```python
from build123d import *

# Parameters (mm, degrees)
BOSS_EXTRUDE1_DEPTH          = 4
BOSS_EXTRUDE1_DEPTH_BACK     = 1
SKETCH1_W                    = 120
SKETCH1_H                    = 120
FILLET1_R                    = 2.5
SKETCH34_W                   = 110
SKETCH34_H                   = 110
BOSS_EXTRUDE4_DEPTH          = 5
SKETCH35_W                   = 5
SKETCH35_H                   = 110
BOSS_EXTRUDE5_DEPTH          = 105
SKETCH36_W                   = 90
SKETCH36_H                   = 9.090388829
CUT_EXTRUDE17_DEPTH          = 5
F_97_0_0059_DIAMETER_HOLE2_D = 0.14986
F_1_0MM_DOWEL_HOLE1_D        = 1
SKETCH46_W                   = 17
SKETCH46_H                   = 15
CUT_EXTRUDE23_DEPTH          = 10
SKETCH50_W                   = 17
SKETCH50_H                   = 15
CUT_EXTRUDE24_DEPTH          = 10
SKETCH51_W                   = 17
SKETCH51_H                   = 15
CUT_EXTRUDE25_DEPTH          = 10
SKETCH52_W                   = 17
SKETCH52_H                   = 15
CUT_EXTRUDE26_DEPTH          = 10
SKETCH53_W                   = 0.977162156
SKETCH53_H                   = 13.998719243
BOSS_EXTRUDE6_DEPTH          = 5
SKETCH55_W                   = 2.272024092
SKETCH55_H                   = 13.774773728
CUT_EXTRUDE27_DEPTH          = 5
SKETCH56_W                   = 0.906735868
SKETCH56_H                   = 14
BOSS_EXTRUDE7_DEPTH          = 5
SKETCH57_W                   = 2.385496373
SKETCH57_H                   = 13.848261841
CUT_EXTRUDE28_DEPTH          = 5
SKETCH58_W                   = 0.96928262
SKETCH58_H                   = 13.634621905
BOSS_EXTRUDE8_DEPTH          = 5
SKETCH59_W                   = 2.435671648
SKETCH59_H                   = 13.900580395
CUT_EXTRUDE29_DEPTH          = 5
SKETCH60_W                   = 0.869613575
SKETCH60_H                   = 13.953535455
BOSS_EXTRUDE10_DEPTH         = 5
SKETCH62_W                   = 2.354070132
SKETCH62_H                   = 13.876017007
CUT_EXTRUDE30_DEPTH          = 5
SKETCH63_W                   = 9.117005695
SKETCH63_H                   = 6.066926996
CUT_EXTRUDE33_DEPTH          = 1
SKETCH64_W                   = 9.176846486
SKETCH64_H                   = 5.926214746
CUT_EXTRUDE34_DEPTH          = 1
SKETCH65_W                   = 9.062729826
SKETCH65_H                   = 5.966132982
CUT_EXTRUDE35_DEPTH          = 1
SKETCH67_W                   = 8.803701295
SKETCH67_H                   = 6.022435514
CUT_EXTRUDE36_DEPTH          = 1


with BuildPart() as part:
    # Sketch1 → Boss-Extrude1 (new, two sides: drawn at the far end of the back side and taken through both)
    with BuildSketch(Plane(origin=(0, 0, 0), x_dir=(1, 0, 0), z_dir=(0, 1, 0)).offset(-BOSS_EXTRUDE1_DEPTH_BACK)):
        Rectangle(SKETCH1_W, SKETCH1_H)
    extrude(amount=BOSS_EXTRUDE1_DEPTH + BOSS_EXTRUDE1_DEPTH_BACK)

    # Fillet1
    fillet1_edges = [part.edges().sort_by_distance(p)[0] for p in [
        (-60, 1.5, -60),
        (60, 1.5, -60),
        (60, 1.5, 60),
        (-60, 1.5, 60),
    ]]
    fillet(fillet1_edges, radius=FILLET1_R)

    # Sketch34 → Boss-Extrude4 (add)
    with BuildSketch(Plane(origin=(0, 4, 0), x_dir=(1, 0, 0), z_dir=(0, 1, 0))):
        Rectangle(SKETCH34_W, SKETCH34_H)
    extrude(amount=BOSS_EXTRUDE4_DEPTH)

    # Sketch35 → Boss-Extrude5 (add)
    with BuildSketch(Plane(origin=(0, 9, 0), x_dir=(1, 0, 0), z_dir=(0, 1, 0))):
        with Locations((-12.5, 0)):
            Rectangle(SKETCH35_W, SKETCH35_H)
    extrude(amount=BOSS_EXTRUDE5_DEPTH)

    # Sketch36 → Cut-Extrude17 (cut)
    with BuildSketch(Plane(origin=(-15, 5, 0), x_dir=(0, 0, 1), z_dir=(-1, 0, 0))):
        with Locations((0, 19.545194415)):
            Rectangle(SKETCH36_W, SKETCH36_H)
    extrude(amount=-CUT_EXTRUDE17_DEPTH, mode=Mode.SUBTRACT)

    # 97 _0.0059_ Diameter Hole2 (through all)
    with Locations(Plane(origin=(0, -1, 0), x_dir=(-1, 0, 0), z_dir=(0, -1, 0))):
        with Locations((57.307733748, 57.378842828), (-57.10337646, 57.378842828), (-57.10337646, -56.921022458), (57.307733748, -56.921022458)):
            Hole(F_97_0_0059_DIAMETER_HOLE2_D / 2)

    # 1.0mm Dowel Hole1 (through all)
    with Locations(Plane(origin=(0, -1, 0), x_dir=(-1, 0, 0), z_dir=(0, -1, 0))):
        with Locations((57.307733748, -56.846092458), (-57.10337646, -56.921022458), (-57.10337646, 57.378842828), (57.307733748, 57.378842828)):
            Hole(F_1_0MM_DOWEL_HOLE1_D / 2)

    # Sketch46 → Cut-Extrude23 (cut)
    with BuildSketch(Plane(origin=(0, -1, 4), x_dir=(1, 0, 0), z_dir=(0, -1, 0))):
        with Locations((17.5, 31.9)):
            Rectangle(SKETCH46_W, SKETCH46_H)
    extrude(amount=-CUT_EXTRUDE23_DEPTH, mode=Mode.SUBTRACT)

    # Sketch50 → Cut-Extrude24 (cut)
    with BuildSketch(Plane(origin=(0, -1, 5), x_dir=(-1, 0, 0), z_dir=(0, -1, 0))):
        with Locations((-17.5, -7)):
            Rectangle(SKETCH50_W, SKETCH50_H)
    extrude(amount=-CUT_EXTRUDE24_DEPTH, mode=Mode.SUBTRACT)

    # Sketch51 → Cut-Extrude25 (cut)
    with BuildSketch(Plane(origin=(0, -1, 6), x_dir=(-1, 0, 0), z_dir=(0, -1, 0))):
        with Locations((-17.5, 18)):
            Rectangle(SKETCH51_W, SKETCH51_H)
    extrude(amount=-CUT_EXTRUDE25_DEPTH, mode=Mode.SUBTRACT)

    # Sketch52 → Cut-Extrude26 (cut)
    with BuildSketch(Plane(origin=(0, -1, 4), x_dir=(1, 0, 0), z_dir=(0, -1, 0))):
        with Locations((17.5, -43)):
            Rectangle(SKETCH52_W, SKETCH52_H)
    extrude(amount=-CUT_EXTRUDE26_DEPTH, mode=Mode.SUBTRACT)

    # Sketch53 → Boss-Extrude6 (add)
    with BuildSketch(Plane(origin=(-2.93050065, 9, 0.122093772), x_dir=(1, 0, 0), z_dir=(0, 1, 0))):
        with Locations((29.779301797, 39.085351217)):
            Rectangle(SKETCH53_W, SKETCH53_H)
    extrude(amount=BOSS_EXTRUDE6_DEPTH)

    # Sketch55 → Cut-Extrude27 (cut)
    with BuildSketch(Plane(origin=(-2.539176839, 9, 0.049591215), x_dir=(1, 0, 0), z_dir=(0, 1, 0))):
        with Locations((31.467069737, 39.084159637)):
            Rectangle(SKETCH55_W, SKETCH55_H)
    extrude(amount=-CUT_EXTRUDE27_DEPTH, mode=Mode.SUBTRACT)

    # Sketch56 → Boss-Extrude7 (add)
    with BuildSketch(Plane(origin=(-2.001675953, 9, 0), x_dir=(1, 0, 0), z_dir=(0, 1, 0))):
        with Locations((28.881264054, 12)):
            Rectangle(SKETCH56_W, SKETCH56_H)
    extrude(amount=BOSS_EXTRUDE7_DEPTH)

    # Sketch57 → Cut-Extrude28 (cut)
    with BuildSketch(Plane(origin=(-2.324919513, 9, 0), x_dir=(1, 0, 0), z_dir=(0, 1, 0))):
        with Locations((31.20631194, 12.028513798)):
            Rectangle(SKETCH57_W, SKETCH57_H)
    extrude(amount=-CUT_EXTRUDE28_DEPTH, mode=Mode.SUBTRACT)

    # Sketch58 → Boss-Extrude8 (add)
    with BuildSketch(Plane(origin=(-1.839703038, 9, 0), x_dir=(1, 0, 0), z_dir=(0, 1, 0))):
        with Locations((28.596634058, -11.879280286)):
            Rectangle(SKETCH58_W, SKETCH58_H)
    extrude(amount=BOSS_EXTRUDE8_DEPTH)

    # Sketch59 → Cut-Extrude29 (cut)
    with BuildSketch(Plane(origin=(-2.765819175, 9, 0), x_dir=(1, 0, 0), z_dir=(0, 1, 0))):
        with Locations((31.546866825, -11.916750925)):
            Rectangle(SKETCH59_W, SKETCH59_H)
    extrude(amount=-CUT_EXTRUDE29_DEPTH, mode=Mode.SUBTRACT)

    # Sketch60 → Boss-Extrude10 (add)
    with BuildSketch(Plane(origin=(-1.803689022, 9, -0.186210488), x_dir=(1, 0, 0), z_dir=(0, 1, 0))):
        with Locations((28.551773242, -36.1181464)):
            Rectangle(SKETCH60_W, SKETCH60_H)
    extrude(amount=BOSS_EXTRUDE10_DEPTH)

    # Sketch62 → Cut-Extrude30 (cut)
    with BuildSketch(Plane(origin=(-2.856074078, 9, -0.042608941), x_dir=(1, 0, 0), z_dir=(0, 1, 0))):
        with Locations((31.403731497, -36.065246957)):
            Rectangle(SKETCH62_W, SKETCH62_H)
    extrude(amount=-CUT_EXTRUDE30_DEPTH, mode=Mode.SUBTRACT)

    # Sketch63 → Cut-Extrude33 (cut)
    with BuildSketch(Plane(origin=(9, 0, 0), x_dir=(0, 0, -1), z_dir=(1, 0, 0))):
        with Locations((-35.854544031, 5.966536502)):
            Rectangle(SKETCH63_W, SKETCH63_H)
    extrude(amount=-CUT_EXTRUDE33_DEPTH, mode=Mode.SUBTRACT)

    # Sketch64 → Cut-Extrude34 (cut)
    with BuildSketch(Plane(origin=(9, 0, 0), x_dir=(0, 0, -1), z_dir=(1, 0, 0))):
        with Locations((-11.959924601, 6.036892627)):
            Rectangle(SKETCH64_W, SKETCH64_H)
    extrude(amount=-CUT_EXTRUDE34_DEPTH, mode=Mode.SUBTRACT)

    # Sketch65 → Cut-Extrude35 (cut)
    with BuildSketch(Plane(origin=(9, 0.251826278, 0.170802287), x_dir=(0, 0, -1), z_dir=(1, 0, 0))):
        with Locations((12.086740933, 6.016933509)):
            Rectangle(SKETCH65_W, SKETCH65_H)
    extrude(amount=-CUT_EXTRUDE35_DEPTH, mode=Mode.SUBTRACT)

    # Sketch67 → Cut-Extrude36 (cut)
    with BuildSketch(Plane(origin=(9, 0, 0), x_dir=(0, 0, -1), z_dir=(1, 0, 0))):
        with Locations((38.763636035, 5.988782243)):
            Rectangle(SKETCH67_W, SKETCH67_H)
    extrude(amount=-CUT_EXTRUDE36_DEPTH, mode=Mode.SUBTRACT)


solid = part.part
```
Work out the finished part from the listing and answer in its coordinate system (mm). A direction names the side the tool comes from. Give positions to 0.01 mm unless a question says otherwise; leave off trailing zeros. Write each loop counter-clockwise with the first axis right and the second up, starting at its lowest first coordinate (ties: lowest second). Pieces come first, ordered by that corner, then holes. Notation, with made-up numbers: (53.5, 57.25) -> (77.5, 57.25) arc R21 ccw to (77.5, 71.25) -> close; hole circle Ø8 at (-12, -33). An arc over 180 degrees is marked (long way). Write item = value, one per line.
Q1. Flat-ended cylindrical pins translate along their axes: pin 1 Ø0.8 at (x, y) = (8.5, 7) entering from -Z; pin 2 Ø1.1 at (x, z) = (8.5, 14) entering from +Y; pin 3 Ø0.8 at (x, y) = (8.5, 5) entering from +Z. Find the tip coordinate at first contact, or state that the pin passes through.
Computed values:
pin_1 = -55
pin_2 = 9
pin_3 = 55
Q2. Section C-C on x = 51 is taken. Determine the outline of the cut face in (y, z), and give its area (3 significant figures).
Computed values:
outline = (-1, -60) -> (4, -60) -> (4, -55) -> (9, -55) -> (9, 55) -> (4, 55) -> (4, 60) -> (-1, 60) -> close
area = 1,150 mm^2
Q3. Consider line 1 along X through (y, z) = (6, 39.5); line 2 along Y through (x, z) = (7, -39.5); line 3 along X through (y, z) = (56, -17.5). Determine where each line is inside the solid, lowest interval first.
Computed values:
line_1 = -55 to 8, 26 to 27.37, 29.72 to 55
line_2 = -1 to 9
line_3 = -15 to -10
Q4. Section A-A on z = 13.5 is taken. State how many separate pieces and enclosed holes the cut face has, and give its area (3 significant figures).
Computed values:
separate_pieces = 3
enclosed_holes = 0
area = 1,450 mm^2
Q5. A tool of negligible diameter and unlimited length cuts with its end or side. For faces 4 (the flat face through (27.689, 7, -12)), 5 (the flat face through (26.272, 11, 12)), 6 (the flat face through (27.183, 11, 36)), 7 (the flat face through (9, 2.8, -39.1)), from which of +Z, -Z, +X, -X, +Y, -Y can it reach the whole face along a straight path? Write none if from no direction.
Computed values:
face_4 = +Y
face_5 = +Z, -Z, +Y
face_6 = +Z, +X, +Y
face_7 = +Y, -Y
Q6. Section B-B on z = -2 is taken. Determine the outline of the cut face in (x, y), and give its area (3 significant figures).
Computed values:
outline = (-60, -1) -> (60, -1) -> (60, 4) -> (55, 4) -> (55, 9) -> (-10, 9) -> (-10, 20) -> (-15, 20) -> (-15, 9) -> (-55, 9) -> (-55, 4) -> (-60, 4) -> close; (-15, 29.09) -> (-10, 29.09) -> (-10, 114) -> (-15, 114) -> close
area = 1,630 mm^2
Q7. For a pull along Y with two mould halves and no side action, classify faces 1 (the flat face through (-13, 24, -45)), 2 (the flat face through (17, 4, 28.4)), 3 (the flat face through (-1, -1, -1)) as pulls with the +Y half, pulls with the -Y half, needs draft (parallel to the pull), parting line crosses it, or undercut.
Computed values:
face_1 = undercut
face_2 = needs draft
face_3 = pulls with the -Y half
